Can you work these out from the model? Positions are in its coordinate system, mm. A direction names the side the tool comes from. Give positions to 0.01 mm unless a question says otherwise; leave off trailing zeros. Write each loop counter-clockwise with the first axis right and the second up, starting at its lowest first coordinate (ties: lowest second). Pieces come first, ordered by that corner, then holes. Notation, with made-up numbers: M 18.5,-29.5 L 59.5,-29.5 A26 ccw 59.5,-9.5 Z; hole C -25.5,46 d3. An arc over 180 degrees is marked long. Write each question's results on one line, items separated by ' | '.
Autodesk Inventor part; units mm, degrees
ref_plane "YZ Plane" through (0, 0, 0) normal (1, 0, 0) x (0, 1, 0)
ref_plane "XZ Plane" through (0, 0, 0) normal (0, 1, 0) x (-1, 0, 0)
ref_plane "XY Plane" through (0, 0, 0) normal (0, 0, 1) x (1, 0, 0)
sketch "Sketch1" plane through (0, 0, 0) normal (0, 0, 1) x (1, 0, 0)
  line L0 (0, 23.4) -> (0, -35.4)
  line L1 (-58.1, 0) -> (58.1, 0)
  line L2 (-10, 15) -> (10, 15)
  line L3 (10, 15) -> (10, -15)
  line L4 (10, -15) -> (-10, -15)
  line L5 (-10, -15) -> (-10, 15)
  line L6 (-41.5, -15) -> (41.5, -15)
  line L7 (41.5, -15) -> (41.5, -27)
  line L8 (41.5, -27) -> (-41.5, -27)
  line L9 (-41.5, -27) -> (-41.5, -15)
  point P0 (0, 0)
  point P1 (10, -15)
  point P2 (-10, -15)
  dimension "d0" = 30
  dimension "d1" = 12
  dimension "d2" = 83
  dimension "d3" = 20
extrude "Extrusion1" add sketch "Sketch1" along normal blind 12
sketch "Sketch2" plane through (41.5, -27, 0) normal (1, 0, 0) x (0, 0, -1)
  line L0 (0, 12) -> (-12, 12)
  line L1 (-12, 0) -> (-12, 12)
  point P0 (0, 27)
  point P1 (-6, 6)
  dimension "d6" = 6
  dimension "d7" = 6
hole "Hole1" at (41.5, -21, 6) direction (-1, 0, 0) diameter 6.647 depth 35 tip angle 118
sketch "Sketch3" plane through (-41.5, -27, 0) normal (-1, 0, 0) x (0, 0, 1)
  line L0 (0, 12) -> (12, 12)
  line L1 (0, 12) -> (0, 0)
  point P0 (0, 27)
  point P1 (6, 6)
  dimension "d15" = 6
  dimension "d16" = 6
hole "Hole2" at (-41.5, -21, 6) direction (1, 0, 0) diameter 6.647 depth 35 tip angle 118
sketch "Sketch4" plane through (0, 0, 12) normal (0, 0, 1) x (1, 0, 0)
  line L0 (-10, 15) -> (-10, -15)
  line L1 (-10, -15) -> (-41.5, -15)
  line L2 (-41.5, -15) -> (-41.5, -27)
  line L3 (-41.5, -27) -> (41.5, -27)
  line L4 (41.5, -27) -> (41.5, -15)
  line L5 (41.5, -15) -> (10, -15)
  line L6 (10, -15) -> (10, 15)
  circle A0 centre (0, -10) radius 2
  line L7 (10, 15) -> (-10, 15)
  circle A1 centre (0, -4) radius 2
  circle A2 centre (0, 2) radius 2
  circle A3 centre (0, 8) radius 2
  point P0 (0, 0)
  dimension "d26" = 4
  dimension "d50" = 17
  dimension "d51" = 10
  dimension "d52" = 4
  dimension "d53" = 6
  dimension "d54" = 4
  dimension "d55" = 10
  dimension "d56" = 6
  dimension "d57" = 10
  dimension "d58" = 4
  dimension "d59" = 10
  dimension "d60" = 6
extrude "Extrusion2" cut sketch "Sketch4" against normal through all contours A0 | A1 | A2 | A3
fillet "Fillet2" radius 5 2 edges at (10, -15, 6) (-10, -15, 6)
sketch "Sketch5" plane through (0, 0, 12) normal (0, 0, 1) x (1, 0, 0)
  line L0 (-10, 15) -> (-10, -10)
  arc A0 (-15, -15) -> (-10, -10) centre (-15, -10) ccw
  line L1 (-15, -15) -> (-41.5, -15)
  line L2 (-41.5, -15) -> (-41.5, -27)
  line L3 (-41.5, -27) -> (41.5, -27)
  line L4 (41.5, -27) -> (41.5, -15)
  line L5 (41.5, -15) -> (15, -15)
  arc A1 (10, -10) -> (15, -15) centre (15, -10) ccw
  line L6 (10, -10) -> (10, 15)
  circle A2 centre (0, -10) radius 2
  line L7 (-54.6159, 30) -> (65.6495, 30)
  line L8 (0, 98.4) -> (0, -47.9)
  circle A3 centre (0, 30) radius 45
  line L9 (10, 15) -> (-10, 15)
  circle A4 centre (0, 8) radius 2
  point P0 (0, 0)
  point P1 (-11.4484, -13.5194)
  point P2 (11.4484, -13.5194)
  point P3 (10.181, -11.3332)
  point P4 (-10.181, -11.3332)
  dimension "d42" = 57
  dimension "d43" = 90
extrude "Extrusion3" cut sketch "Sketch5" against normal blind 6 contours L9 L8 A4 A2 A3 A0 L0 | L0 A0 A3 L7 L8 L9 | L9 L6 A1 A3 L8 A2 A4 | L8 L7 A3 A1 L6 L9 | L8 A3 L7 | L7 A3 L8 | A4 L8 | L8 A4
fillet "Fillet4" radius 10 2 edges at (10, 15, 3) (-10, 15, 3)
properties part number "workTrianglePc1"
Item 1: I want a section at B-B, the plane z = 10.25. Please give me the cut outline in (x, y).
Geometry says:
outline: M -41.5,-27 L 41.5,-27 L 41.5,-15 L 15,-15 A5 cw 11.45,-13.52 A45 cw -11.45,-13.52 A5 cw -15,-15 L -41.5,-15 Z
Item 2: I'm going to push flat-ended pins straight in: pin 1 (6 mm diameter, centred on x = -29.5, z = 4, fed in from +Y); pin 2 (3 mm diameter, centred on y = -4.5, z = 3, fed in from +X); pin 3 (1.5 mm diameter, centred on y = -8, z = 2.5, fed in from -X). Where does each tip first touch, or does it pass through?
Geometry says:
pin 1: stops at y = -15 | pin 2: stops at x = 10 | pin 3: stops at x = -10
Item 3: Thinking about a two-plate mould opening in Z: for faces 5 (the face through (1, -27, 6)), 6 (the face through (-1, -20, 12)), 7 (the face through (23.8, -24.3, 6.4)), which applies, +Z half, -Z half, draft (parallel to the pull), parting line (faces both ways), or undercut?
Geometry says:
face 5: draft | face 6: +Z half | face 7: undercut
Item 4: If I drill on line 1 (Y direction, x = 0, z = 2.55); line 2 (Z direction, x = -20, y = -21); line 3 (X direction, y = -10, z = 2.05), over which ranges is the centre line in solid material (lowest first)? Write a range as from..to.
Geometry says:
line 1: y = -27..-12, -8..-6, -2..0, 4..6, 10..15 | line 2: z = 0..2.68, 9.32..12 | line 3: x = -10..-2, 2..10
Item 5: I want a section at A-A, the plane y = 2. Please give me the cut outline in (x, z), and give its area (3 significant figures).
Geometry says:
outline: M -10,0 L -2,0 L -2,6 L -10,6 Z; M 2,0 L 10,0 L 10,6 L 2,6 Z | area: 96.0 mm2
Item 6: For faces 1 (the face through (-28, -15, 6)), 2 (the face through (0, -15, 9)), 3 (the face through (10, -2, 3)), 4 (the face through (-23.8, -24.3, 5.6)), which set-ups out of +Z, -Z, +X, -X, +Y, -Y let a thin tool reach every point of the face, with its end or its side?
Geometry says:
face 1: +Z, -Z, -X, +Y | face 2: +Z, +Y | face 3: +Z, -Z, +X, +Y | face 4: -X
Item 7: I want a section at C-C, the plane x = 23.5. Please give me the cut outline in (y, z).
Geometry says:
outline: M -27,0 L -15,0 L -15,12 L -27,12 Z; hole C -21,6 d6.65
